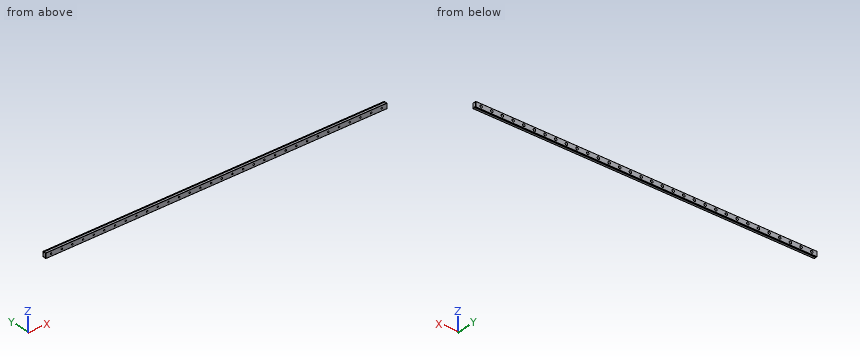
```python
from build123d import *

# Parameters (mm, degrees)
SKETCH1_W           = 12
SKETCH1_H           = 8
BOSS_EXTRUDE1_DEPTH = 800
SKETCH2_R           = 3
CUT_EXTRUDE1_DEPTH  = 4.5
SKETCH3_R           = 1.75
CUT_EXTRUDE2_DEPTH  = 3.5
CUT_EXTRUDE3_REACH  = 802.032
SKETCH4_W           = 1.75
SKETCH4_H           = 0.5
FILLET2_R           = 0.4


with BuildPart() as part:
    # Sketch1 → Boss-Extrude1 (new body)
    with BuildSketch(Plane(origin=(0, 0, 0), x_dir=(0, 0, -1), z_dir=(1, 0, 0))):
        Rectangle(SKETCH1_W, SKETCH1_H)
    extrude(amount=BOSS_EXTRUDE1_DEPTH)

    # Sketch2 → Cut-Extrude1 (cut)
    with BuildSketch(Plane(origin=(0, 4, 0), x_dir=(1, 0, 0), z_dir=(0, 1, 0))):
        with Locations(Location((412.5, 0, 0), (0, 0, 270))):
            Circle(SKETCH2_R)
        with Locations(Location((437.5, 0, 0), (0, 0, 270))):
            Circle(SKETCH2_R)
        with Locations(Location((462.5, 0, 0), (0, 0, 270))):
            Circle(SKETCH2_R)
        with Locations(Location((487.5, 0, 0), (0, 0, 270))):
            Circle(SKETCH2_R)
        with Locations(Location((512.5, 0, 0), (0, 0, 270))):
            Circle(SKETCH2_R)
        with Locations(Location((537.5, 0, 0), (0, 0, 270))):
            Circle(SKETCH2_R)
        with Locations(Location((562.5, 0, 0), (0, 0, 270))):
            Circle(SKETCH2_R)
        with Locations(Location((587.5, 0, 0), (0, 0, 270))):
            Circle(SKETCH2_R)
        with Locations(Location((612.5, 0, 0), (0, 0, 270))):
            Circle(SKETCH2_R)
        with Locations(Location((637.5, 0, 0), (0, 0, 270))):
            Circle(SKETCH2_R)
        with Locations(Location((662.5, 0, 0), (0, 0, 270))):
            Circle(SKETCH2_R)
        with Locations(Location((687.5, 0, 0), (0, 0, 270))):
            Circle(SKETCH2_R)
        with Locations(Location((712.5, 0, 0), (0, 0, 270))):
            Circle(SKETCH2_R)
        with Locations(Location((737.5, 0, 0), (0, 0, 270))):
            Circle(SKETCH2_R)
        with Locations(Location((762.5, 0, 0), (0, 0, 270))):
            Circle(SKETCH2_R)
        with Locations(Location((787.5, 0, 0), (0, 0, 270))):
            Circle(SKETCH2_R)
        with Locations(Location((387.5, 0, 0), (0, 0, 270))):
            Circle(SKETCH2_R)
        with Locations(Location((362.5, 0, 0), (0, 0, 270))):
            Circle(SKETCH2_R)
        with Locations(Location((337.5, 0, 0), (0, 0, 270))):
            Circle(SKETCH2_R)
        with Locations(Location((312.5, 0, 0), (0, 0, 270))):
            Circle(SKETCH2_R)
        with Locations(Location((287.5, 0, 0), (0, 0, 270))):
            Circle(SKETCH2_R)
        with Locations(Location((262.5, 0, 0), (0, 0, 270))):
            Circle(SKETCH2_R)
        with Locations(Location((237.5, 0, 0), (0, 0, 270))):
            Circle(SKETCH2_R)
        with Locations(Location((212.5, 0, 0), (0, 0, 270))):
            Circle(SKETCH2_R)
        with Locations(Location((187.5, 0, 0), (0, 0, 270))):
            Circle(SKETCH2_R)
        with Locations(Location((162.5, 0, 0), (0, 0, 270))):
            Circle(SKETCH2_R)
        with Locations(Location((137.5, 0, 0), (0, 0, 270))):
            Circle(SKETCH2_R)
        with Locations(Location((112.5, 0, 0), (0, 0, 270))):
            Circle(SKETCH2_R)
        with Locations(Location((87.5, 0, 0), (0, 0, 270))):
            Circle(SKETCH2_R)
        with Locations(Location((62.5, 0, 0), (0, 0, 270))):
            Circle(SKETCH2_R)
        with Locations(Location((37.5, 0, 0), (0, 0, 270))):
            Circle(SKETCH2_R)
        with Locations(Location((12.5, 0, 0), (0, 0, 270))):
            Circle(SKETCH2_R)
    extrude(amount=-CUT_EXTRUDE1_DEPTH, mode=Mode.SUBTRACT)

    # Sketch3 → Cut-Extrude2 (cut)
    with BuildSketch(Plane(origin=(0, -0.5, 0), x_dir=(1, 0, 0), z_dir=(0, 1, 0))):
        with Locations(Location((12.5, 0, 0), (0, 0, 270))):
            Circle(SKETCH3_R)
        with Locations(Location((37.5, 0, 0), (0, 0, 270))):
            Circle(SKETCH3_R)
        with Locations(Location((62.5, 0, 0), (0, 0, 270))):
            Circle(SKETCH3_R)
        with Locations(Location((87.5, 0, 0), (0, 0, 270))):
            Circle(SKETCH3_R)
        with Locations(Location((112.5, 0, 0), (0, 0, 270))):
            Circle(SKETCH3_R)
        with Locations(Location((137.5, 0, 0), (0, 0, 270))):
            Circle(SKETCH3_R)
        with Locations(Location((162.5, 0, 0), (0, 0, 270))):
            Circle(SKETCH3_R)
        with Locations(Location((187.5, 0, 0), (0, 0, 270))):
            Circle(SKETCH3_R)
        with Locations(Location((212.5, 0, 0), (0, 0, 270))):
            Circle(SKETCH3_R)
        with Locations(Location((237.5, 0, 0), (0, 0, 270))):
            Circle(SKETCH3_R)
        with Locations(Location((262.5, 0, 0), (0, 0, 270))):
            Circle(SKETCH3_R)
        with Locations(Location((287.5, 0, 0), (0, 0, 270))):
            Circle(SKETCH3_R)
        with Locations(Location((312.5, 0, 0), (0, 0, 270))):
            Circle(SKETCH3_R)
        with Locations(Location((337.5, 0, 0), (0, 0, 270))):
            Circle(SKETCH3_R)
        with Locations(Location((362.5, 0, 0), (0, 0, 270))):
            Circle(SKETCH3_R)
        with Locations(Location((387.5, 0, 0), (0, 0, 270))):
            Circle(SKETCH3_R)
        with Locations(Location((412.5, 0, 0), (0, 0, 270))):
            Circle(SKETCH3_R)
        with Locations(Location((437.5, 0, 0), (0, 0, 270))):
            Circle(SKETCH3_R)
        with Locations(Location((462.5, 0, 0), (0, 0, 270))):
            Circle(SKETCH3_R)
        with Locations(Location((487.5, 0, 0), (0, 0, 270))):
            Circle(SKETCH3_R)
        with Locations(Location((512.5, 0, 0), (0, 0, 270))):
            Circle(SKETCH3_R)
        with Locations(Location((537.5, 0, 0), (0, 0, 270))):
            Circle(SKETCH3_R)
        with Locations(Location((562.5, 0, 0), (0, 0, 270))):
            Circle(SKETCH3_R)
        with Locations(Location((587.5, 0, 0), (0, 0, 270))):
            Circle(SKETCH3_R)
        with Locations(Location((612.5, 0, 0), (0, 0, 270))):
            Circle(SKETCH3_R)
        with Locations(Location((637.5, 0, 0), (0, 0, 270))):
            Circle(SKETCH3_R)
        with Locations(Location((662.5, 0, 0), (0, 0, 270))):
            Circle(SKETCH3_R)
        with Locations(Location((687.5, 0, 0), (0, 0, 270))):
            Circle(SKETCH3_R)
        with Locations(Location((712.5, 0, 0), (0, 0, 270))):
            Circle(SKETCH3_R)
        with Locations(Location((737.5, 0, 0), (0, 0, 270))):
            Circle(SKETCH3_R)
        with Locations(Location((762.5, 0, 0), (0, 0, 270))):
            Circle(SKETCH3_R)
        with Locations(Location((787.5, 0, 0), (0, 0, 270))):
            Circle(SKETCH3_R)
    extrude(amount=-CUT_EXTRUDE2_DEPTH, mode=Mode.SUBTRACT)

    # Sketch4 → Cut-Extrude3 (cut, up to next)
    with BuildSketch(Plane.ZY, mode=Mode.PRIVATE) as cut_extrude3_sk1:
        with Locations((-5.125, 1.75)):
            Rectangle(SKETCH4_W, SKETCH4_H)
    cut_extrude3_tool1 = extrude(cut_extrude3_sk1.sketch, amount=-CUT_EXTRUDE3_REACH, mode=Mode.PRIVATE) & part.part
    # Sketch4 → Cut-Extrude3 (cut, up to next)
    with BuildSketch(Plane.ZY, mode=Mode.PRIVATE) as cut_extrude3_sk2:
        with Locations((5.125, 1.75)):
            Rectangle(SKETCH4_W, SKETCH4_H)
    cut_extrude3_tool2 = extrude(cut_extrude3_sk2.sketch, amount=-CUT_EXTRUDE3_REACH, mode=Mode.PRIVATE) & part.part
    add(cut_extrude3_tool1.solids().sort_by_distance((0, 1.75, -5.125))[0], mode=Mode.SUBTRACT)
    add(cut_extrude3_tool2.solids().sort_by_distance((0, 1.75, 5.125))[0], mode=Mode.SUBTRACT)

    # Fillet2
    fillet2_edges = [part.edges().sort_by_distance(p)[0] for p in [
        (800, -1.25, -6),
        (800, 4, 0),
        (0, 3, -6),
        (800, 3, -6),
        (400, 1.5, -6),
        (800, 2, -5.125),
        (400, 2, -6),
        (800, 1.75, -4.25),
        (800, 1.5, -5.125),
        (0, 1.5, -5.125),
        (0, 1.75, -4.25),
        (0, 2, -5.125),
        (0, -1.25, 6),
        (800, -1.25, 6),
        (800, 1.5, 5.125),
        (400, 1.5, 6),
        (800, 1.75, 4.25),
        (800, 2, 5.125),
        (400, 2, 6),
        (0, 1.5, 5.125),
        (0, 2, 5.125),
        (0, 1.75, 4.25),
        (800, 3, 6),
        (0, 4, 0),
        (0, -1.25, -6),
        (0, -4, 0),
        (0, 3, 6),
        (800, -4, 0),
        (400, 4, 6),
        (400, 4, -6),
        (400, -4, -6),
        (400, -4, 6),
    ]]
    fillet(fillet2_edges, radius=FILLET2_R)


solid = part.part
```
Model file for the job. Use its own axes, mm. Give positions to 0.01 mm unless a question says otherwise; leave off trailing zeros. Write each loop counter-clockwise with the first axis right and the second up, starting at its lowest first coordinate (ties: lowest second). Pieces come first, ordered by that corner, then holes. Notation, with made-up numbers: (-18.5, 6) - (-12.5, 6) arc R27 ccw to (-12.5, 44) - close; hole circle Ø5 at (22.25, 51.25). An arc over 180 degrees is marked (long way). One line per question, with ' | ' between items. Start each with the question number.
(1) Slice it at A-A on x = 150.5. Write the cut outline in (y, z), plus the area to 3 significant figures.
(2) Wall check: line 1 along Y through (x, z) = (731, 5); line 2 along Z through (x, y) = (487.5, 2.35); line 3 along Z through (x, y) = (662.5, -1.2). Give the ranges that are in metal, low to high. Write a range as from..to.
(3) Pin check, flat tip, straight feed: P1, Ø3, axis at x = 488.5, z = 0.5, coming from the +Y side. Stop position of the tip, or through.
Results below:
1) outline: (-4, -5.6) arc R0.4 ccw to (-3.6, -6) - (1.1, -6) arc R0.4 ccw to (1.5, -5.6) - (1.5, -4.25) - (2, -4.25) - (2, -5.6) arc R0.4 ccw to (2.4, -6) - (3.6, -6) arc R0.4 ccw to (4, -5.6) - (4, 5.6) arc R0.4 ccw to (3.6, 6) - (2.4, 6) arc R0.4 ccw to (2, 5.6) - (2, 4.25) - (1.5, 4.25) - (1.5, 5.6) arc R0.4 ccw to (1.1, 6) - (-3.6, 6) arc R0.4 ccw to (-4, 5.6) - close | area: 94.0 mm^2
2) line 1: -4..1.5, 2..4 | line 2: -6..-3, 3..6 | line 3: -6..-1.75, 1.75..6
3) P1: y = -0.5
